Work out the finished part from the listing and answer in its coordinate system (mm). Face numbers are marked on the shaded views. A direction names the side the tool comes from. Coordinates: 2 decimals unless noted, no trailing zeros. Write each loop counter-clockwise with the first axis right and the second up, starting at its lowest first coordinate (ties: lowest second). Pieces come first, ordered by that corner, then holes. Notation, with made-up numbers: (20, -40) - (40, -40) arc R24 ccw to (40, -19) - close; hole circle Ø3 at (-9, -13.5). An arc over 180 degrees is marked (long way). Answer as a JSON object with one key per item and string values. Group by question number.
from build123d import *

# Parameters (mm, degrees)
CROQUIS1_W              = 45
CROQUIS1_H              = 45
SALIENTE_EXTRUIR1_DEPTH = 2
CORTAR_EXTRUIR1_DEPTH   = 2
CROQUIS3_W              = 45
CROQUIS3_H              = 4
SALIENTE_EXTRUIR2_DEPTH = 120
CROQUIS4_W              = 45
CROQUIS4_H              = 4
SALIENTE_EXTRUIR3_DEPTH = 3
CROQUIS5_W              = 45
CROQUIS5_H              = 3
SALIENTE_EXTRUIR4_DEPTH = 45
CROQUIS6_R              = 12
CROQUIS6_R_2            = 2
CORTAR_EXTRUIR2_DEPTH   = 3
CROQUIS7_W              = 45
CROQUIS7_H              = 3
SALIENTE_EXTRUIR5_DEPTH = 45
CROQUIS8_R              = 12
CROQUIS8_R_2            = 2
CORTAR_EXTRUIR4_DEPTH   = 44
CROQUIS11_W             = 27.899668072
CROQUIS11_H             = 7
CORTAR_EXTRUIR5_DEPTH   = 45
SALIENTE_EXTRUIR6_DEPTH = 1
SALIENTE_EXTRUIR7_DEPTH = 1
SALIENTE_EXTRUIR8_DEPTH = 1


with BuildPart() as part:
    # Croquis1 → Saliente-Extruir1 (new body)
    with BuildSketch(Plane(origin=(0, 0, 0), x_dir=(1, 0, 0), z_dir=(0, 1, 0))):
        Rectangle(CROQUIS1_W, CROQUIS1_H)
    extrude(amount=SALIENTE_EXTRUIR1_DEPTH)

    # Croquis2 → Cortar-Extruir1 (cut)
    with BuildSketch(Plane(origin=(0, 2, 0), x_dir=(1, 0, 0), z_dir=(0, 1, 0))):
        with BuildLine():
            Line((-18, -14.692077551), (-18, 15.307922449))
            ThreePointArc((-18, 15.307922449), (-15, 18.307922449), (-12, 15.307922449))
            Line((-12, 15.307922449), (-12, -14.692077551))
            ThreePointArc((-12, -14.692077551), (-15, -17.692077551), (-18, -14.692077551))
        make_face()
        with BuildLine():
            Line((18, -14.692077551), (18, 15.307922449))
            ThreePointArc((18, 15.307922449), (15, 18.307922449), (12, 15.307922449))
            Line((12, 15.307922449), (12, -14.692077551))
            ThreePointArc((12, -14.692077551), (15, -17.692077551), (18, -14.692077551))
        make_face()
    extrude(amount=-CORTAR_EXTRUIR1_DEPTH, mode=Mode.SUBTRACT)

    # Croquis3 → Saliente-Extruir2 (add)
    with BuildSketch(Plane(origin=(0, 2, 0), x_dir=(1, 0, 0), z_dir=(0, 1, 0))):
        with Locations((0, -20.5)):
            Rectangle(CROQUIS3_W, CROQUIS3_H)
    extrude(amount=SALIENTE_EXTRUIR2_DEPTH)

    # Croquis4 → Saliente-Extruir3 (add)
    with BuildSketch(Plane(origin=(0, 122, 0), x_dir=(1, 0, 0), z_dir=(0, 1, 0))):
        with Locations((0, -20.5)):
            Rectangle(CROQUIS4_W, CROQUIS4_H)
    extrude(amount=SALIENTE_EXTRUIR3_DEPTH)

    # Croquis5 → Saliente-Extruir4 (add)
    with BuildSketch(Plane.XY.offset(22.5)):
        with Locations((0, 123.5)):
            Rectangle(CROQUIS5_W, CROQUIS5_H)
    extrude(amount=SALIENTE_EXTRUIR4_DEPTH)

    # Croquis6 → Cortar-Extruir2 (cut)
    with BuildSketch(Plane(origin=(0, 125, 0), x_dir=(1, 0, 0), z_dir=(0, 1, 0))):
        with Locations((0, -43)):
            Circle(CROQUIS6_R)
        with Locations((-15.5, -27.5)):
            Circle(CROQUIS6_R_2)
        with Locations((15.5, -27.5)):
            Circle(CROQUIS6_R_2)
        with Locations((15.5, -58.5)):
            Circle(CROQUIS6_R_2)
        with Locations((-15.5, -58.5)):
            Circle(CROQUIS6_R_2)
    extrude(amount=-CORTAR_EXTRUIR2_DEPTH, mode=Mode.SUBTRACT)

    # Croquis7 → Saliente-Extruir5 (add)
    with BuildSketch(Plane.XY.offset(22.5)):
        with Locations((0, 82.5)):
            Rectangle(CROQUIS7_W, CROQUIS7_H)
    extrude(amount=SALIENTE_EXTRUIR5_DEPTH)

    # Croquis8 → Cortar-Extruir4 (cut)
    with BuildSketch(Plane(origin=(0, 125, 0), x_dir=(1, 0, 0), z_dir=(0, 1, 0))):
        with Locations((0, -43)):
            Circle(CROQUIS8_R)
        with Locations((15.5, -58.5)):
            Circle(CROQUIS8_R_2)
        with Locations((15.5, -27.5)):
            Circle(CROQUIS8_R_2)
        with Locations((-15.5, -27.5)):
            Circle(CROQUIS8_R_2)
        with Locations((-15.5, -58.5)):
            Circle(CROQUIS8_R_2)
    extrude(amount=-CORTAR_EXTRUIR4_DEPTH, mode=Mode.SUBTRACT)

    # Croquis11 → Cortar-Extruir5 (cut)
    with BuildSketch(Plane(origin=(0, 84, 0), x_dir=(1, 0, 0), z_dir=(0, 1, 0))):
        with Locations((-22.5, -43)):
            Rectangle(CROQUIS11_W, CROQUIS11_H)
    extrude(amount=-CORTAR_EXTRUIR5_DEPTH, mode=Mode.SUBTRACT)

    # Croquis14 → Saliente-Extruir6 (add)
    with BuildSketch(Plane(origin=(22.5, 0, 0), x_dir=(0, 0, -1), z_dir=(1, 0, 0))):
        Polygon((-67.5, 122), (-67.5, 84), (-18.5, 84), (-18.5, 125), (-67.5, 125), align=None)
    extrude(amount=-SALIENTE_EXTRUIR6_DEPTH)

    # Croquis16 → Saliente-Extruir7 (add)
    with BuildSketch(Plane(origin=(22.5, 0, 0), x_dir=(0, 0, -1), z_dir=(1, 0, 0))):
        Polygon((-18.5, 125), (22.5, 2), (22.5, 0), (-22.5, 0), (-22.5, 125), align=None)
    extrude(amount=-SALIENTE_EXTRUIR7_DEPTH)

    # Croquis17 → Saliente-Extruir8 (add)
    with BuildSketch(Plane(origin=(22.5, 0, 0), x_dir=(0, 0, -1), z_dir=(1, 0, 0))):
        Polygon((-67.5, 81), (-22.5, 0), (-22.5, 84), (-67.5, 84), align=None)
    extrude(amount=-SALIENTE_EXTRUIR8_DEPTH)


solid = part.part
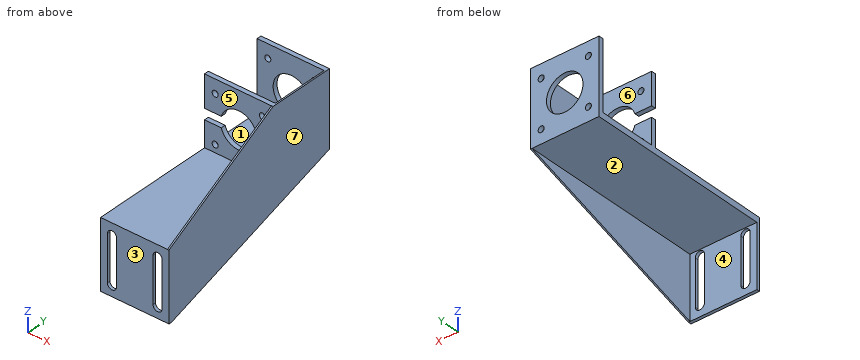
Q1. Section C-C on x = -6 is taken. Determine the outline of the cut face in (y, z).
Q2. Section B-B on z = -5 is taken. Determine the outline of the cut face in (x, y), plus the area to 4 significant figures.
Q3. For a pull along Y with two mould halves and no side action, classify the marked faces 1, 2 and 3 as +Y half, -Y half, draft (parallel to the pull), parting line (faces both ways), or undercut.
Q4. A tool of negligible diameter and unlimited length cuts with its end or side. For the marked faces 4, 5, 6 and 7, from which of +Z, -Z, +X, -X, +Y, -Y can it reach the whole face along a straight path? Write none if from no direction.
Q5. Section A-A on z = 58.5 is taken. Determine the outline of the cut face in (x, y), plus the area to 3 significant figures.
Q6. Section D-D on x = 15.5 is taken. Count the separate pieces of the cut face and the enclosed holes in it, plus the area to 3 significant figures.
Q7. Consider L1, parallel to Z at x = -15.5, y = 123.75; L2, parallel to X at y = 124.2, z = 27.5; L3, parallel to Z at x = -15.5, y = 82.55. Determine where each line is inside the solid, lowest interval first. Write a range as from..to.
Q8. Flat-ended cylindrical pins translate along their axes: pin 1 Ø12 at (x, y) = (2, 89.5) entering from +Z; pin 2 Ø12 at (x, y) = (-11.5, 44) entering from -Z; pin 3 Ø22 at (x, y) = (-7.5, 41.5) entering from +Z; pin 4 Ø3.5 at (x, z) = (-15.5, 58.5) entering from -Y. Find the tip coordinate at first contact, or state that the pin passes through.
Numbers:
{
 "1": {"outline": "(0, -22.5) - (2, -22.5) - (2, 18.5) - (125, 18.5) - (125, 32.61) - (122, 32.61) - (122, 22.5) - (84, 22.5) - (84, 32.61) - (81, 32.61) - (81, 22.5) - (0, 22.5) - close; (81, 53.39) - (84, 53.39) - (84, 67.5) - (81, 67.5) - close; (122, 53.39) - (125, 53.39) - (125, 67.5) - (122, 67.5) - close"},
 "2": {"outline": "(-22.5, 0) - (-18, 0) - (-18, 2) - (-22.5, 2) - close; (-12, 0) - (12, 0) - (12, 2) - (-12, 2) - close; (18, 0) - (22.5, 0) - (22.5, 54.5) - (21.5, 54.5) - (21.5, 2) - (18, 2) - close", "area": "118.5 mm²"},
 "3": {"face 1": "undercut", "face 2": "draft", "face 3": "-Y half"},
 "4": {"face 4": "-Z, -X, +Y", "face 5": "+Z, -X, -Y", "face 6": "+Z, -X", "face 7": "+Z, -Z, +X, +Y, -Y"},
 "5": {"outline": "(-22.5, 81) - (-17.5, 81) - (-17.5, 84) - (-22.5, 84) - close; (-22.5, 122) - (-17.5, 122) - (-17.5, 125) - (-22.5, 125) - close; (-13.5, 81) - (13.5, 81) - (13.5, 84) - (-13.5, 84) - close; (-13.5, 122) - (13.5, 122) - (13.5, 125) - (-13.5, 125) - close; (17.5, 81) - (21.5, 81) - (21.5, 64.8) - (22.5, 64.8) - (22.5, 125) - (17.5, 125) - (17.5, 122) - (21.5, 122) - (21.5, 84) - (17.5, 84) - close", "area": "276 mm²"},
 "6": {"separate pieces": "6", "enclosed holes": "0", "area": "732 mm²"},
 "7": {"L1": "z = 18.5..25.5, 29.5..56.5, 60.5..67.5", "L2": "x = -22.5..-17.5, -13.5..13.5, 17.5..22.5", "L3": "z = 18.5..25.5, 29.5..39.5, 46.5..56.5, 60.5..67.5"},
 "8": {"pin 1": "stops at z = 67.5", "pin 2": "stops at z = 18.5", "pin 3": "stops at z = 22.5", "pin 4": "passes through"}
}
